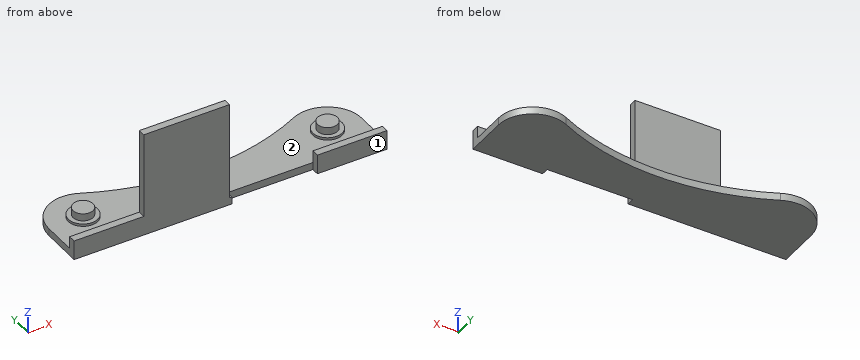
Autodesk Fusion 360 part; units mm, degrees
sketch "Sketch1" plane through (0, 0, 0) normal (0, 0, 1) x (1, 0, 0)
  circle A0 centre (-50, 0) radius 4.1
  circle A1 centre (50, 0) radius 4.1
  circle A2 centre (50, 0) radius 14
  circle A3 centre (50, 0) radius 6
  circle A4 centre (-50, 0) radius 14
  circle A5 centre (-50, 0) radius 6
  line L0 (-64, -14) -> (64, -14)
  line L1 (-64, 0) -> (-64, -14)
  line L2 (64, 0) -> (64, -14)
  arc A6 (-43.8635, 12.5835) -> (43.8635, 12.5835) centre (0, 102.5297) ccw
  line L3 (-64, -14) -> (64, -14)
  line L4 (64, -14) -> (64, -17)
  line L5 (64, -17) -> (-64, -17)
  line L6 (-64, -17) -> (-64, -14)
  line L7 (0.5, -14) -> (35.5, -14)
  line L8 (35.5, -14) -> (35.5, -17)
  line L9 (35.5, -17) -> (0.5, -17)
  line L10 (0.5, -17) -> (0.5, -14)
  line L11 (-0.5, -14) -> (-35.5, -14)
  line L12 (-35.5, -14) -> (-35.5, -17)
  line L13 (-35.5, -17) -> (-0.5, -17)
  line L14 (-0.5, -17) -> (-0.5, -14)
  point P0 (-0.113, 2.4581)
  dimension "d1" = 8.2
  dimension "d2" = 8.2
  dimension "d3" = 50
  dimension "d4" = 50
  dimension "d5" = 28
  dimension "d6" = 12
  dimension "d7" = 28
  dimension "d8" = 12
  dimension "d9" = 14
  dimension "d10" = 3
  dimension "d11" = 3
  dimension "d12" = 35
  dimension "d13" = 35.5
  dimension "d20" = 35
  dimension "d21" = 35.5
extrude "Extrude1" add sketch "Sketch1" against normal blind 3 contours A0 | A1 | A2 | A2 L0 L2 L3 | A2 A4 L0 A6 L3 L7 L11 | L0 L3 L4 L5 L8 | A4 | A4 L0 L1 L3 | L0 L3 L5 L10 L14 | L0 L3 L5 L6 L12 | L0 L3 L5 L11 L12 L13 L14 | A3 | A5
extrude "Extrude2" add sketch "Sketch1" along normal blind 1 contours A3 | A5
extrude "Extrude3" add sketch "Sketch1" along normal blind 4 contours A0 | A1
extrude "Extrude4" add sketch "Sketch1" along normal blind 40 contours L0 L3 L5 L11 L12 L13 L14
extrude "Extrude5" add sketch "Sketch1" along normal blind 5 contours L0 L3 L4 L5 L8 | L0 L3 L5 L6 L12
Model file for the job. Use its own axes, mm. Face numbers are marked on the shaded views. Coordinates: 2 decimals unless noted, no trailing zeros. Order: outer loops, then holes, each group sorted by start corner. A loop starts at its lowest first (then second) coordinate and runs counter-clockwise, first axis right, second up. Notation, with made-up numbers: (18, 15) - (23, 15) arc R21 ccw to (23, 32) - close; hole circle Ø1 at (26.5, -14.75). An arc over 180 degrees is marked (long way). Return JSON: item names as keys, results as strings. Group by question number.
1) Saw through at C-C, the plane z = 13. Write the cut outline in (x, y), plus the area to 3 significant figures.
2) Saw through at D-D, the plane x = 18. Write the cut outline in (y, z), plus the area to 3 significant figures.
3) Flat gauge pins, fed straight in: P1, Ø2.5, axis at x = 19, z = -2, coming from the -Y side; P2, Ø3.5, axis at x = -45, y = -15.5, coming from the +Z side; P3, Ø5, axis at x = -33, z = 13, coming from the +Y side; P4, Ø6, axis at y = -1, z = 2, coming from the +X side. Where does each tip first touch, or does it go through?
4) Mould opens along X. For the marked faces 1 and 2 say: released by +X, released by -X, zero draft, split by the parting line, or undercut.
5) Saw through at A-A, the plane y = 9. Write the cut outline in (x, z), plus the area to 3 significant figures.
6) Probe line 1 (Z direction, x = -17, y = -13.5); line 2 (Y direction, x = -30.5, z = 37.5); line 3 (Z direction, x = -51, y = 5). List the from-to ranges inside material, lowest first. Write a range as from..to.
7) Saw through at B-B, the plane x = 50. Write the cut outline in (y, z), plus the area to 3 significant figures.
Values found:
{
 "1": {"outline": "(-35.5, -17) - (-0.5, -17) - (-0.5, -14) - (-35.5, -14) - close", "area": "105 mm²"},
 "2": {"outline": "(-14, -3) - (4.09, -3) - (4.09, 0) - (-14, 0) - close", "area": "54.3 mm²"},
 "3": {"P1": "stops at y = -14", "P2": "stops at z = 5", "P3": "stops at y = -14", "P4": "stops at x = 64"},
 "4": {"face 1": "zero draft", "face 2": "undercut"},
 "5": {"outline": "(-60.72, -3) - (-35.59, -3) - (-35.59, 0) - (-60.72, 0) - close; (35.59, -3) - (60.72, -3) - (60.72, 0) - (35.59, 0) - close", "area": "151 mm²"},
 "6": {"line 1": "z = -3..0", "line 2": "y = -17..-14", "line 3": "z = -3..1"},
 "7": {"outline": "(-17, -3) - (14, -3) - (14, 0) - (6, 0) - (6, 1) - (4.1, 1) - (4.1, 4) - (-4.1, 4) - (-4.1, 1) - (-6, 1) - (-6, 0) - (-14, 0) - (-14, 5) - (-17, 5) - close", "area": "145 mm²"}
}
